from build123d import *

# Parameters (mm, degrees)
BOSS_EXTRUDE1_DEPTH          = 6.35
BOSS_EXTRUDE2_DEPTH          = 19.05
CUT_EXTRUDE2_START           = -25.4
CUT_EXTRUDE2_DEPTH           = 31.75
CUT_EXTRUDE3_DEPTH           = 147.267687771
BOSS_EXTRUDE3_DEPTH          = 19.05
F_1_4_0_25_DIAMETER_HOLE1_D  = 6.35
F_3_8_0_375_DIAMETER_HOLE1_D = 9.525
F_1_4_20_TAPPED_HOLE1_D      = 5.1054
F_1_4_20_TAPPED_HOLE1_DEPTH  = 16.51
F_1_4_20_TAPPED_HOLE1_TIP    = 1.533816902


with BuildPart() as part:
    # Sketch1 → Boss-Extrude1 (new body)
    with BuildSketch(Plane(origin=(0, 0, 0), x_dir=(1, 0, 0), z_dir=(0, 1, 0))):
        with BuildLine():
            Line((-81.75625, 112.7125), (81.75625, 112.7125))
            ThreePointArc((81.75625, 112.7125), (87.368910076, 110.387660076), (89.69375, 104.775))
            Line((89.69375, 104.775), (89.69375, -87.3125))
            ThreePointArc((89.69375, -87.3125), (82.254262242, -105.273012242), (64.29375, -112.7125))
            Line((64.29375, -112.7125), (-64.29375, -112.7125))
            ThreePointArc((-64.29375, -112.7125), (-82.254262242, -105.273012242), (-89.69375, -87.3125))
            Line((-89.69375, -87.3125), (-89.69375, 104.775))
            ThreePointArc((-89.69375, 104.775), (-87.368910076, 110.387660076), (-81.75625, 112.7125))
        make_face()
    extrude(amount=BOSS_EXTRUDE1_DEPTH)

    # Sketch2 → Boss-Extrude2 (add)
    with BuildSketch(Plane(origin=(0, 6.35, 0), x_dir=(1, 0, 0), z_dir=(0, 1, 0))):
        with BuildLine():
            Line((89.69375, -87.3125), (89.69375, 104.775))
            ThreePointArc((89.69375, 104.775), (87.368910076, 110.387660076), (81.75625, 112.7125))
            Line((81.75625, 112.7125), (-81.75625, 112.7125))
            ThreePointArc((-81.75625, 112.7125), (-87.368910076, 110.387660076), (-89.69375, 104.775))
            Line((-89.69375, 104.775), (-89.69375, -87.3125))
            ThreePointArc((-89.69375, -87.3125), (-82.254262242, -105.273012242), (-64.29375, -112.7125))
            Line((-64.29375, -112.7125), (64.29375, -112.7125))
            ThreePointArc((64.29375, -112.7125), (82.254262242, -105.273012242), (89.69375, -87.3125))
        make_face()
        with BuildLine():
            Line((81.75625, 106.3625), (-81.75625, 106.3625))
            ThreePointArc((-81.75625, 106.3625), (-82.878782015, 105.897532015), (-83.34375, 104.775))
            Line((-83.34375, 104.775), (-83.34375, -87.3125))
            ThreePointArc((-83.34375, -87.3125), (-77.764134182, -100.782884182), (-64.29375, -106.3625))
            Line((-64.29375, -106.3625), (64.29375, -106.3625))
            ThreePointArc((64.29375, -106.3625), (77.764134182, -100.782884182), (83.34375, -87.3125))
            Line((83.34375, -87.3125), (83.34375, 104.775))
            ThreePointArc((83.34375, 104.775), (82.878782015, 105.897532015), (81.75625, 106.3625))
        make_face(mode=Mode.SUBTRACT)
    extrude(amount=BOSS_EXTRUDE2_DEPTH)

    # Sketch7 → Cut-Extrude2 (cut)
    with BuildSketch(Plane(origin=(13.135345572, 31.711529428, 0), x_dir=(0, 0, -1), z_dir=(0.3826834323650874, 0.9238795325112878, 0)).offset(CUT_EXTRUDE2_START)):
        with BuildLine():
            Line((46.94555, -40.046221701), (3.85445, -40.046221701))
            add(Edge.make_bspline(
                [(3.85445, -71.796221701), (-27.89555, -71.796221701), (-27.89555, -40.046221701), (3.85445, -40.046221701)],
                knots=[0, 0, 0, 0, 1, 1, 1, 1], degree=3, weights=[1, 0.333333333, 0.333333333, 1]))
            Line((3.85445, -71.796221701), (46.94555, -71.796221701))
            add(Edge.make_bspline(
                [(46.94555, -40.046221701), (78.69555, -40.046221701), (78.69555, -71.796221701), (46.94555, -71.796221701)],
                knots=[0, 0, 0, 0, 1, 1, 1, 1], degree=3, weights=[1, 0.333333333, 0.333333333, 1]))
        make_face()
    cut_extrude2 = extrude(amount=CUT_EXTRUDE2_DEPTH, mode=Mode.SUBTRACT)

    # Sketch8 → Cut-Extrude3 (cut, through all)
    with BuildSketch(Plane.XZ):
        with BuildLine():
            Line((13.49375, 87.78875), (26.19375, 87.78875))
            ThreePointArc((26.19375, 87.78875), (35.71875, 78.26375), (26.19375, 68.73875))
            Line((26.19375, 68.73875), (13.49375, 68.73875))
            ThreePointArc((13.49375, 68.73875), (3.96875, 78.26375), (13.49375, 87.78875))
        make_face()
        with BuildLine():
            Line((-13.49375, 87.78875), (-26.19375, 87.78875))
            ThreePointArc((-26.19375, 87.78875), (-35.71875, 78.26375), (-26.19375, 68.73875))
            Line((-26.19375, 68.73875), (-13.49375, 68.73875))
            ThreePointArc((-13.49375, 68.73875), (-3.96875, 78.26375), (-13.49375, 87.78875))
        make_face()
    extrude(amount=-CUT_EXTRUDE3_DEPTH, mode=Mode.SUBTRACT)

    # Sketch9 → Boss-Extrude3 (add)
    with BuildSketch(Plane(origin=(0, 6.35, 0), x_dir=(1, 0, 0), z_dir=(0, 1, 0))):
        with BuildLine():
            Line((-81.75625, 106.3625), (-71.120073585, 106.3625))
            ThreePointArc((-71.120073585, 106.3625), (-73.309655038, 105.486708137), (-74.291288385, 103.342489328))
            ThreePointArc((-74.291288385, 103.342489328), (-76.143589924, 99.162339924), (-80.323739328, 97.310038385))
            ThreePointArc((-80.323739328, 97.310038385), (-82.467958137, 96.328405038), (-83.34375, 94.138823585))
            Line((-83.34375, 94.138823585), (-83.34375, 104.775))
            ThreePointArc((-83.34375, 104.775), (-82.878782015, 105.897532015), (-81.75625, 106.3625))
        make_face()
        with BuildLine():
            Line((-9.525, 106.3625), (9.525, 106.3625))
            ThreePointArc((9.525, 106.3625), (7.27993597, 105.43256403), (6.35, 103.1875))
            ThreePointArc((6.35, 103.1875), (0, 96.8375), (-6.35, 103.1875))
            ThreePointArc((-6.35, 103.1875), (-7.27993597, 105.43256403), (-9.525, 106.3625))
        make_face()
        with BuildLine():
            Line((83.34375, 104.775), (83.34375, 94.138823585))
            ThreePointArc((83.34375, 94.138823585), (82.467958137, 96.328405038), (80.323739328, 97.310038385))
            ThreePointArc((80.323739328, 97.310038385), (76.143589924, 99.162339924), (74.291288385, 103.342489328))
            ThreePointArc((74.291288385, 103.342489328), (73.309655038, 105.486708137), (71.120073585, 106.3625))
            Line((71.120073585, 106.3625), (81.75625, 106.3625))
            ThreePointArc((81.75625, 106.3625), (82.878782015, 105.897532015), (83.34375, 104.775))
        make_face()
        with BuildLine():
            ThreePointArc((-83.049421546, -90.648258512), (-81.324581361, -92.941426622), (-78.45534091, -92.907472557))
            ThreePointArc((-78.45534091, -92.907472557), (-71.028942091, -94.047692091), (-69.888722557, -101.47409091))
            ThreePointArc((-69.888722557, -101.47409091), (-69.922676622, -104.343331361), (-67.629508512, -106.068171546))
            ThreePointArc((-67.629508512, -106.068171546), (-77.764134182, -100.782884182), (-83.049421546, -90.648258512))
        make_face()
        with BuildLine():
            ThreePointArc((69.888722557, -101.47409091), (69.922676622, -104.343331361), (67.629508512, -106.068171546))
            ThreePointArc((67.629508512, -106.068171546), (77.764134182, -100.782884182), (83.049421546, -90.648258512))
            ThreePointArc((83.049421546, -90.648258512), (81.324581361, -92.941426622), (78.45534091, -92.907472557))
            ThreePointArc((78.45534091, -92.907472557), (71.028942091, -94.047692091), (69.888722557, -101.47409091))
        make_face()
    extrude(amount=BOSS_EXTRUDE3_DEPTH)

    # 1/4 (0.25) Diameter Hole1 (through all)
    with Locations(Plane(origin=(0, 6.35, 0), x_dir=(1, 0, 0), z_dir=(0, 1, 0))):
        with Locations((-57.94375, 70.96125), (-57.94375, -94.13875), (57.94375, -94.13875), (57.94375, 70.96125)):
            Hole(F_1_4_0_25_DIAMETER_HOLE1_D / 2)

    # 3/8 (0.375) Diameter Hole1 (through all)
    with Locations(Plane(origin=(0, 0, 0), x_dir=(-1, 0, 0), z_dir=(0, -1, 0))):
        with Locations((-73.81875, 77.7875), (73.81875, 77.7875), (73.81875, -74.6125), (-73.81875, -74.6125)):
            Hole(F_3_8_0_375_DIAMETER_HOLE1_D / 2)

    # Mirror1: Cut-Extrude2 across plane
    add(cut_extrude2.mirror(Plane(origin=(0, 0, 0), x_dir=(0, 0, 1), z_dir=(1, 0, 0))), mode=Mode.SUBTRACT)

    # 1/4-20 Tapped Hole1
    with Locations(Plane(origin=(0, 25.4, 0), x_dir=(1, 0, 0), z_dir=(0, 1, 0))):
        with Locations((-75.519070151, -98.537820151), (75.519070151, -98.537820151), (80.633717985, 103.652467985), (0, 103.1875), (-80.633717985, 103.652467985)):
            Hole(F_1_4_20_TAPPED_HOLE1_D / 2, depth=F_1_4_20_TAPPED_HOLE1_DEPTH)
            with Locations((0, 0, -(F_1_4_20_TAPPED_HOLE1_DEPTH + F_1_4_20_TAPPED_HOLE1_TIP / 2))):  # 118° drill point
                Cone(0, F_1_4_20_TAPPED_HOLE1_D / 2, F_1_4_20_TAPPED_HOLE1_TIP, mode=Mode.SUBTRACT)


solid = part.part
Here's how the part is built. I have some questions about the finished solid (model axes, mm). A direction names the side the tool comes from. Round coordinates to 2 decimals unless told otherwise and drop trailing zeros. Write each loop counter-clockwise with the first axis right and the second up, starting at its lowest first coordinate (ties: lowest second). Pieces come first, ordered by that corner, then holes. Notation, with made-up numbers: (-32, 62.25) -> (25, 62.25) arc R13 cw to (25, 70.25) -> close; hole circle Ø4 at (6, 73). An arc over 180 degrees is marked (long way). One line per item, written item: value.
1) If I drill on line 1 (X direction, y = 13.5, z = 58); line 2 (Z direction, x = -13.5, y = 4.25); line 3 (Z direction, x = -41, y = 16.25), over which ranges is the centre line in solid material (lowest first)? Write a range as [from, to].
Filled sheet:
line 1: x = [-89.69, -83.34], [83.34, 89.69]
line 2: z = [-112.71, 68.74], [87.79, 112.71]
line 3: z = [-112.71, -106.36], [106.36, 112.71]
2) For faces 5 (the face through (-72.97, 17.03, 98.43)), 6 (the face through (-89.694, 13, -10)), 7 (the face through (44.642, 3.131, -25.702)), 8 (the face through (-35.716, 3.131, 78.473)), which set-ups out of +Z, -Z, +X, -X, +Y, -Y let a thin tool reach every point of the face, with its end or its side?
Filled sheet:
face 5: +Y
face 6: +Z, -Z, -X, +Y, -Y
face 7: -Y
face 8: +Y, -Y
3) Suppose I cut it at D-D on y = 14. Give the number of separate pieces and of enclosed holes in the cut face, plus the area to 3 significant figures.
Filled sheet:
separate pieces: 1
enclosed holes: 6
area: 5,210 mm2
4) Suppose I cut it at A-A on z = -8. List the corners of the cut face in (x, y) for me, plus the area to 3 significant figures.
Filled sheet:
outline: (-89.69, 0) -> (-77.71, 0) -> (-80.34, 6.35) -> (-83.34, 6.35) -> (-83.34, 25.4) -> (-89.69, 25.4) -> close; (-45.98, 6.35) -> (-43.35, 0) -> (43.35, 0) -> (45.98, 6.35) -> close; (77.71, 0) -> (89.69, 0) -> (89.69, 25.4) -> (83.34, 25.4) -> (83.34, 6.35) -> (80.34, 6.35) -> close
area: 945 mm2
5) I'm going to push flat-ended pins straight in: pin 1 Ø2 at (x, z) = (-51, 21) entering from +Y; pin 2 Ø4.5 at (x, z) = (0, -103.19) entering from +Y; pin 3 Ø11 at (x, z) = (-73.82, 74.61) entering from +Y. Where does each tip first touch, or does it pass through?
Filled sheet:
pin 1: stops at y = 6.35
pin 2: stops at y = 8.71
pin 3: stops at y = 6.35
6) Suppose I cut it at B-B on x = 17. List the corners of the cut face in (y, z) for me, plus the area to 3 significant figures.
Filled sheet:
outline: (0, -112.71) -> (25.4, -112.71) -> (25.4, -106.36) -> (6.35, -106.36) -> (6.35, 68.74) -> (0, 68.74) -> close; (0, 87.79) -> (6.35, 87.79) -> (6.35, 106.36) -> (25.4, 106.36) -> (25.4, 112.71) -> (0, 112.71) -> close
area: 1,550 mm2
7) Suppose I cut it at C-C on z = 66. List the corners of the cut face in (x, y) for me.
Filled sheet:
outline: (-89.69, 0) -> (89.69, 0) -> (89.69, 25.4) -> (83.34, 25.4) -> (83.34, 6.35) -> (-83.34, 6.35) -> (-83.34, 25.4) -> (-89.69, 25.4) -> close
8) We'd pull the mould along X, two halves only. Please class faces 1 (the face through (-86, 25.4, -9)), 2 (the face through (-59.65, 3.13, 91.46)), 3 (the face through (82.056, 12.522, 105.469)), 4 (the face through (69.94, 15.74, 104.31)): released by +X, released by -X, zero draft, split by the parting line, or undercut.
Filled sheet:
face 1: zero draft
face 2: undercut
face 3: released by +X
face 4: undercut
